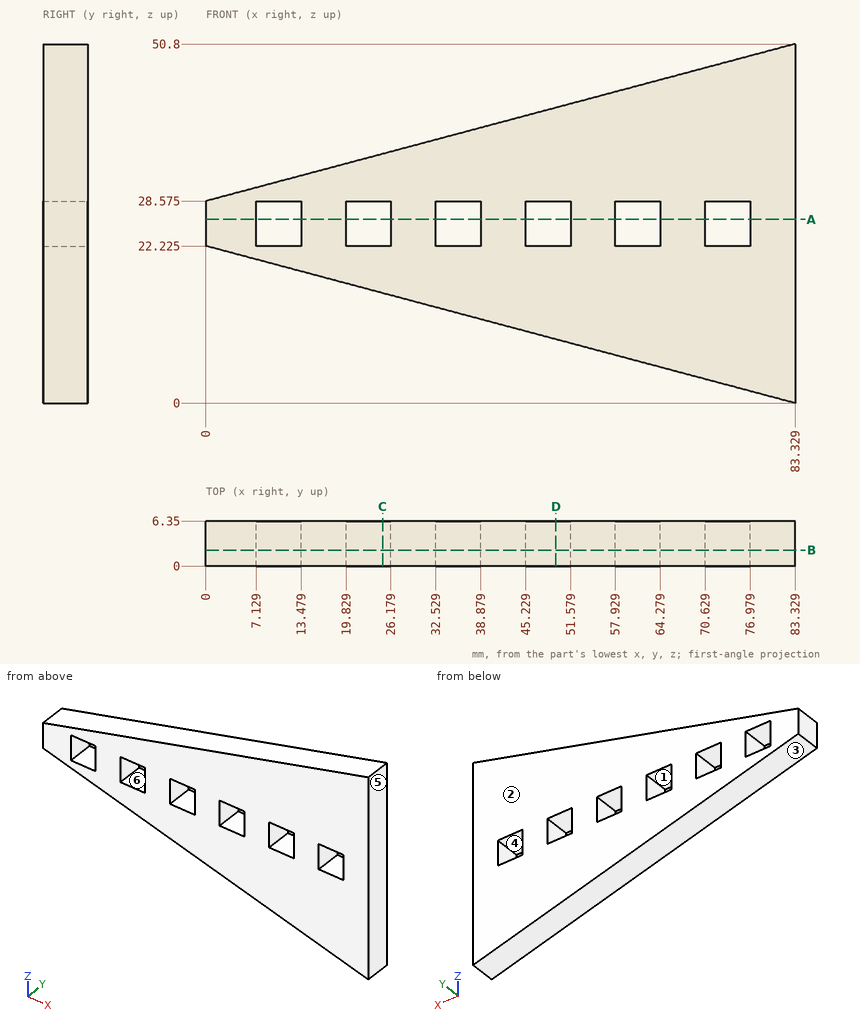
Print and shaded views of the part. All mm, measured from the part's lowest x, y and z. A direction names the side the tool comes from. Round coordinates to 2 decimals unless told otherwise and drop trailing zeros. Write each loop counter-clockwise with the first axis right and the second up, starting at its lowest first coordinate (ties: lowest second). Pieces come first, ordered by that corner, then holes. Notation, with made-up numbers: (70, -13) -> (124, -13) arc R21 ccw to (124, 24) -> close; hole circle Ø2 at (25, 72). An arc over 180 degrees is marked (long way). Return JSON: item names as keys, results as strings. Group by question number.
Q1. Saw through at B-B on y = 2.25. Write the cut outline in (x, z) (3 decimals).
Q2. Saw through at A-A on z = 26. Write the cut outline in (x, y), plus the area to 3 significant figures.
Q3. Which spindle directions (+Z, -Z, +X, -X, +Y, -Y) get a long thin tool onto all of the face, cutting with end or side? Do the marked faces 1 and 2. Say none if no direction does.
Q4. Saw through at C-C on x = 25. Write the cut outline in (y, z) (3 decimals), plus the area to 3 significant figures.
Q5. Pin check, flat tips, straight feed: pin 1 (2 mm diameter, centred on x = 42.5, y = 3.5, fed in from -Z); pin 2 (1.9 mm diameter, centred on x = 62, y = 2.5, fed in from +Z); pin 3 (1.9 mm diameter, centred on x = 36.5, y = 2.5, fed in from +Z). Stop position of each tip, or through.
Q6. Saw through at D-D on x = 49.5. Write the cut outline in (y, z) (3 decimals).
Q7. Mould opens along Z. For the marked faces 3, 4, 5 and 6 say: pulls with the +Z half, pulls with the -Z half, needs draft (parallel to the pull), parting line crosses it, or undercut.
Q8. Probe L1, parallel to Z at x = 25, y = 4 (3 decimals); L2, parallel to Z at x = 23, y = 5.5 (3 decimals); L3, parallel to Z at x = 65, y = 4. List the from-to ranges inside material, lowest first. Write a range as [from, to].
Answer:
{
 "1": {"outline": "(0, 22.225) -> (83.329, 0) -> (83.329, 50.8) -> (0, 28.575) -> close; hole (7.129, 22.225) -> (13.479, 22.225) -> (13.479, 28.575) -> (7.129, 28.575) -> close; hole (19.829, 22.225) -> (26.179, 22.225) -> (26.179, 28.575) -> (19.829, 28.575) -> close; hole (32.529, 22.225) -> (38.879, 22.225) -> (38.879, 28.575) -> (32.529, 28.575) -> close; hole (45.229, 22.225) -> (51.579, 22.225) -> (51.579, 28.575) -> (45.229, 28.575) -> close; hole (57.929, 22.225) -> (64.279, 22.225) -> (64.279, 28.575) -> (57.929, 28.575) -> close; hole (70.629, 22.225) -> (76.979, 22.225) -> (76.979, 28.575) -> (70.629, 28.575) -> close"},
 "2": {"outline": "(0, 0) -> (7.13, 0) -> (7.13, 6.35) -> (0, 6.35) -> close; (13.48, 0) -> (19.83, 0) -> (19.83, 6.35) -> (13.48, 6.35) -> close; (26.18, 0) -> (32.53, 0) -> (32.53, 6.35) -> (26.18, 6.35) -> close; (38.88, 0) -> (45.23, 0) -> (45.23, 6.35) -> (38.88, 6.35) -> close; (51.58, 0) -> (57.93, 0) -> (57.93, 6.35) -> (51.58, 6.35) -> close; (64.28, 0) -> (70.63, 0) -> (70.63, 6.35) -> (64.28, 6.35) -> close; (76.98, 0) -> (83.33, 0) -> (83.33, 6.35) -> (76.98, 6.35) -> close", "area": "287 mm2"},
 "3": {"face 1": "+Y, -Y", "face 2": "+Z, -Z, +X, -X, +Y"},
 "4": {"outline": "(0, 15.557) -> (6.35, 15.557) -> (6.35, 22.225) -> (0, 22.225) -> close; (0, 28.575) -> (6.35, 28.575) -> (6.35, 35.243) -> (0, 35.243) -> close", "area": "84.7 mm2"},
 "5": {"pin 1": "z = 10.62", "pin 2": "z = 45.36", "pin 3": "z = 38.56"},
 "6": {"outline": "(0, 9.023) -> (6.35, 9.023) -> (6.35, 22.225) -> (0, 22.225) -> close; (0, 28.575) -> (6.35, 28.575) -> (6.35, 41.777) -> (0, 41.777) -> close"},
 "7": {"face 3": "pulls with the -Z half", "face 4": "undercut", "face 5": "needs draft", "face 6": "undercut"},
 "8": {"L1": "[15.557, 22.225], [28.575, 35.243]", "L2": "[16.091, 22.225], [28.575, 34.709]", "L3": "[4.89, 45.91]"}
}
